Design review of the part built by this model. Coordinates are the model's own, in mm. A direction names the side the tool comes from. Give positions to 0.01 mm unless a question says otherwise; leave off trailing zeros. Order: outer loops, then holes, each group sorted by start corner. A loop starts at its lowest first (then second) coordinate and runs counter-clockwise, first axis right, second up. Notation, with made-up numbers: M 29,49 L 50,49 A22 ccw 50,75 Z; hole C 1,52 d10. An arc over 180 degrees is marked long. Answer as a JSON object with one key per item and string values.
Autodesk Inventor part; units mm, degrees
ref_plane "YZ Plane" through (0, 0, 0) normal (1, 0, 0) x (0, 1, 0)
ref_plane "XZ Plane" through (0, 0, 0) normal (0, 1, 0) x (-1, 0, 0)
ref_plane "XY Plane" through (0, 0, 0) normal (0, 0, 1) x (1, 0, 0)
sketch "Sketch1" plane through (0, 0, 0) normal (0, 1, 0) x (-1, 0, 0)
  line L0 (0, 0) -> (10.5, 0) construction
  line L1 (10.5, -6.0622) -> (0, -12.1244)
  line L2 (0, -12.1244) -> (-10.5, -6.0622)
  line L3 (-10.5, -6.0622) -> (-10.5, 6.0622)
  line L4 (-10.5, 6.0622) -> (0, 12.1244)
  line L5 (0, 12.1244) -> (10.5, 6.0622)
  line L6 (10.5, 6.0622) -> (10.5, -6.0622)
  circle A0 centre (0, 0) radius 7
  dimension "d0" = 10.5
  dimension "d1" = 14
extrude "Extrusion1" add sketch "Sketch1" along normal blind 4
thread "Thread1"
chamfer "Chamfer1" distance 1 angle 45 6 edges at (10.5, 2, 6.0622) (10.5, 2, -6.0622) (0, 2, -12.1244) (-10.5, 2, -6.0622) (-10.5, 2, 6.0622) (0, 2, 12.1244)
chamfer "Chamfer2" distance 1 angle 45 6 edges at (-10.067, 0, -5.8122) (0, 0, -11.6244) (-10.067, 0, 5.8122) (10.067, 0, -5.8122) (10.067, 0, 5.8122) (0, 0, 11.6244)
sketch "Sketch2" plane through (0, 4, 0) normal (0, 1, 0) x (1, 0, 0)
  circle A0 centre (0, 10.1244) radius 0.5
  line L0 (-0.866, 11.6244) -> (0.866, 11.6244)
  circle A1 centre (-8.7679, -5.0622) radius 0.5
  circle A2 centre (8.7679, -5.0622) radius 0.5
  point P0 (0, 0)
  dimension "d12" = 1
  dimension "d13" = 1.5
  dimension "d16" = 360
extrude "Extrusion2" cut sketch "Sketch2" against normal blind 2
sketch "Sketch3" plane through (0, 0, 0) normal (0, -1, 0) x (1, 0, 0)
  circle A0 centre (0, 0) radius 8.5
  dimension "d20" = 17
extrude "Extrusion3" cut sketch "Sketch3" against normal blind 0.1
properties part number "nut"
(1) To check wall thickness, follow L1, parallel to Z at x = 0, y = 3.2; L2, parallel to X at y = 0.15, z = 0; L3, parallel to Y at x = -6.5, z = 3.75. State the ranges of each line that lie inside material, in increasing order. Write a range as from..to.
Checked values:
{"L1": "z = -11.62..-10.62, -9.62..-7, 7..11.62", "L2": "x = -10.5..-7, 7..10.5", "L3": "y = 0.1..4"}
(2) We need section D-D (x = -4.5). Write out the cut boundary in (y, z).
Checked values:
{"outline": "M 0,-9.53 L 4,-9.53 L 4,-5.36 L 0.1,-5.36 L 0.1,-7.21 L 0,-7.21 Z; M 0,7.21 L 0.1,7.21 L 0.1,5.36 L 4,5.36 L 4,9.53 L 0,9.53 Z"}
(3) We need section A-A (x = 0). Write out the cut boundary in (y, z), plus the area to 3 significant figures.
Checked values:
{"outline": "M 0,-10.62 L 1,-11.62 L 4,-11.62 L 4,-10.62 L 2,-10.62 L 2,-9.62 L 4,-9.62 L 4,-7 L 0.1,-7 L 0.1,-8.5 L 0,-8.5 Z; M 0,8.5 L 0.1,8.5 L 0.1,7 L 4,7 L 4,11.62 L 1,11.62 L 0,10.62 Z", "area": "33.7 mm^2"}
(4) Insertion check: pin 1 (2 mm diameter, centred on x = 6, y = 3.5, fed in from -Z); pin 2 (1.5 mm diameter, centred on x = -3, z = 4.5, fed in from +Y). Each pin has a flat end and moves straight along its axis. Give the tip position at first contact, or say it passes through.
Checked values:
{"pin 1": "stops at z = -9.24", "pin 2": "passes through"}
(5) Draft analysis for pull direction Z (two halves, no side actions). For faces 1 (the flat face through (-10.5, 2, 0)), 2 (the flat face through (0, 2, -10)), 3 (the flat face through (-9.53, 0.4, -5.54)), state which applies: +Z half, -Z half, draft (parallel to the pull), parting line (faces both ways), or undercut.
Checked values:
{"face 1": "draft", "face 2": "undercut", "face 3": "-Z half"}
(6) We need section C-C (y = 3.55). Write out the cut boundary in (x, z).
Checked values:
{"outline": "M -10.5,-5.06 L -9.63,-6.56 L -0.87,-11.62 L 0.87,-11.62 L 9.63,-6.56 L 10.5,-5.06 L 10.5,5.06 L 9.63,6.56 L 0.87,11.62 L -0.87,11.62 L -9.63,6.56 L -10.5,5.06 Z; hole C -8.77,5.06 d1; hole C 0,0 d14; hole C 0,-10.12 d1; hole C 8.77,5.06 d1"}
(7) We need section B-B (z = 0). Write out the cut boundary in (x, y).
Checked values:
{"outline": "M -10.5,0 L -8.5,0 L -8.5,0.1 L -7,0.1 L -7,4 L -10.5,4 Z; M 7,0.1 L 8.5,0.1 L 8.5,0 L 10.5,0 L 10.5,4 L 7,4 Z"}
(8) Tool access review of faces 4 (the flat face through (10.5, 2, 0)), 5 (the cylindrical face through (-8.306, 3.014, 5.254)), 6 (the flat face through (2, 0.1, 7)): name each direction out of +Z, -Z, +X, -X, +Y, -Y from which nothing blocks a thin tool from reaching the whole face with its end or side.
Checked values:
{"face 4": "+Z, -Z, +X, +Y, -Y", "face 5": "+Y", "face 6": "-Y"}
